```python
from build123d import *

# Parameters (mm, degrees)
RESSALTO_EXTRUS_O1_DEPTH = 12
RESSALTO_EXTRUS_O3_DEPTH = 6
ESBO_O4_W                = 3
ESBO_O4_H                = 26
RESSALTO_EXTRUS_O4_DEPTH = 22
ESBO_O6_W                = 2.5
ESBO_O6_H                = 9.5
RESSALTO_EXTRUS_O5_DEPTH = 2
ESBO_O7_R                = 1.1
CORTE_EXTRUS_O1_DEPTH    = 55.490824916
ESBO_O8_R                = 28.014084507
ESBO_O8_R_2              = 25.514084507
CORTE_EXTRUS_O2_DEPTH    = 3
FILETE1_R                = 1


with BuildPart() as part:
    # Esboço1 → Ressalto-extrusão1 (new body)
    with BuildSketch(Plane(origin=(0, 0, 0), x_dir=(1, 0, 0), z_dir=(0, 1, 0))):
        with BuildLine():
            Line((1.5, -16.431676725), (1.5, -13))
            Line((1.5, -13), (-0.5, -13))
            Line((-0.5, -13), (-0.5, 13))
            Line((-0.5, 13), (1.5, 13))
            Line((1.5, 13), (1.5, 16.431676725))
            ThreePointArc((1.5, 16.431676725), (6.342987532, 15.232088142), (10.60599556, 12.639733311))
            Line((10.60599556, 12.639733311), (13.819933608, 16.469955527))
            ThreePointArc((13.819933608, 16.469955527), (-21.5, 0), (13.819933608, -16.469955527))
            Line((13.819933608, -16.469955527), (10.60599556, -12.639733311))
            ThreePointArc((10.60599556, -12.639733311), (6.342987532, -15.232088142), (1.5, -16.431676725))
        make_face()
    extrude(amount=-RESSALTO_EXTRUS_O1_DEPTH)

    # Esboço3 → Ressalto-extrusão3 (add)
    with BuildSketch(Plane(origin=(0, 0, 0), x_dir=(1, 0, 0), z_dir=(0, 1, 0))):
        with BuildLine():
            Line((13.819933608, -16.469955527), (22.818960144, -27.194577731))
            ThreePointArc((22.818960144, -27.194577731), (-35.5, 0), (22.818960144, 27.194577731))
            Line((22.818960144, 27.194577731), (13.819933608, 16.469955527))
            ThreePointArc((13.819933608, 16.469955527), (-21.5, 0), (13.819933608, -16.469955527))
        make_face()
    extrude(amount=-RESSALTO_EXTRUS_O3_DEPTH)

    # Esboço4 → Ressalto-extrusão4 (add)
    with BuildSketch(Plane(origin=(0, 0, 0), x_dir=(1, 0, 0), z_dir=(0, 1, 0))):
        with Locations((-2, 0)):
            Rectangle(ESBO_O4_W, ESBO_O4_H)
    extrude(amount=RESSALTO_EXTRUS_O4_DEPTH)

    # Esboço6 → Ressalto-extrusão5 (add)
    with BuildSketch(Plane(origin=(-0.5, 0, 0), x_dir=(0, 0, -1), z_dir=(1, 0, 0))):
        with Locations((-11.75, -7.25)):
            Rectangle(ESBO_O6_W, ESBO_O6_H)
        with Locations((11.75, -7.25)):
            Rectangle(ESBO_O6_W, ESBO_O6_H)
    extrude(amount=RESSALTO_EXTRUS_O5_DEPTH)

    # Esboço7 → Corte-extrusão1 (cut, through all)
    with BuildSketch(Plane(origin=(-0.5, 0, 0), x_dir=(0, 0, -1), z_dir=(1, 0, 0))):
        with Locations((-10.4, 19.5)):
            Circle(ESBO_O7_R)
        with Locations((10.4, 19.5)):
            Circle(ESBO_O7_R)
        with Locations((10.4, 7)):
            Circle(ESBO_O7_R)
        with Locations((-10.4, 7)):
            Circle(ESBO_O7_R)
    extrude(amount=-CORTE_EXTRUS_O1_DEPTH, mode=Mode.SUBTRACT)

    # Esboço8 → Corte-extrusão2 (cut)
    with BuildSketch(Plane(origin=(0, 0, 0), x_dir=(1, 0, 0), z_dir=(0, 1, 0))):
        Circle(ESBO_O8_R)
        Circle(ESBO_O8_R_2, mode=Mode.SUBTRACT)
    extrude(amount=-CORTE_EXTRUS_O2_DEPTH, mode=Mode.SUBTRACT)

    # Filete1
    # the kernel refuses this fillet: 1 mm, written as the material it takes off along each edge
    with BuildSketch(Plane(origin=(-2.5, 21, 12), x_dir=(0, 0, 1), z_dir=(-1, 0, 0))) as filete1_piece_1_section:
        Polygon((0, 0), (FILETE1_R * 1.02, 0), (FILETE1_R * 1.02, FILETE1_R * 1.02), (0, FILETE1_R * 1.02), align=None)
    filete1_piece_1 = extrude(amount=FILETE1_R * 1.02, mode=Mode.PRIVATE)
    filete1_piece_1 = filete1_piece_1 - Plane(origin=(-2.5, 21, 12), x_dir=(0, -0.7071067811865475, -0.7071067811865475), z_dir=(-1, 0, 0)) * Sphere(FILETE1_R, mode=Mode.PRIVATE)
    add(filete1_piece_1, mode=Mode.SUBTRACT)
    with BuildSketch(Plane(origin=(-1.5, 21, 12), x_dir=(0, 0, 1), z_dir=(0, 1, 0))) as filete1_piece_2_section:
        Polygon((0, 0), (FILETE1_R * 1.02, 0), (FILETE1_R * 1.02, FILETE1_R * 1.02), (0, FILETE1_R * 1.02), align=None)
    filete1_piece_2 = extrude(amount=FILETE1_R * 1.02, mode=Mode.PRIVATE)
    filete1_piece_2 = filete1_piece_2 - Plane(origin=(-1.5, 21, 12), x_dir=(-0.7071067811865476, 0, -0.7071067811865475), z_dir=(0, 1, 0)) * Sphere(FILETE1_R, mode=Mode.PRIVATE)
    add(filete1_piece_2, mode=Mode.SUBTRACT)
    with BuildSketch(Plane(origin=(-1.5, 21, -12), x_dir=(1, 0, 0), z_dir=(0, 1, 0))) as filete1_piece_3_section:
        Polygon((0, 0), (FILETE1_R * 1.02, 0), (FILETE1_R * 1.02, FILETE1_R * 1.02), (0, FILETE1_R * 1.02), align=None)
    filete1_piece_3 = extrude(amount=FILETE1_R * 1.02, mode=Mode.PRIVATE)
    filete1_piece_3 = filete1_piece_3 - Plane(origin=(-1.5, 21, -12), x_dir=(-0.7071067811865475, 0, 0.7071067811865477), z_dir=(0, 1, 0)) * Sphere(FILETE1_R, mode=Mode.PRIVATE)
    add(filete1_piece_3, mode=Mode.SUBTRACT)
    with BuildSketch(Plane(origin=(-2.5, 21, -12), x_dir=(0, 1, 0), z_dir=(-1, 0, 0))) as filete1_piece_4_section:
        Polygon((0, 0), (FILETE1_R * 1.02, 0), (FILETE1_R * 1.02, FILETE1_R * 1.02), (0, FILETE1_R * 1.02), align=None)
    filete1_piece_4 = extrude(amount=FILETE1_R * 1.02, mode=Mode.PRIVATE)
    filete1_piece_4 = filete1_piece_4 - Plane(origin=(-2.5, 21, -12), x_dir=(0, -0.7071067811865475, 0.7071067811865475), z_dir=(-1, 0, 0)) * Sphere(FILETE1_R, mode=Mode.PRIVATE)
    add(filete1_piece_4, mode=Mode.SUBTRACT)
    with BuildSketch(Plane(origin=(1.5, 0, -10.5), x_dir=(-1, 0, 0), z_dir=(0, 0, -1))) as filete1_piece_5_section:
        with BuildLine():
            CenterArc((FILETE1_R, -FILETE1_R), FILETE1_R, 90, 90)
            Line((0, -FILETE1_R), (0, 0))
            Line((0, 0), (FILETE1_R, 0))
        make_face()
    filete1_piece_5 = extrude(amount=8.431676725, mode=Mode.PRIVATE)
    filete1_piece_5 = filete1_piece_5 & Plane(origin=(0, 0, 0), x_dir=(0.09090909090909027, 0, -0.9958591954639385), z_dir=(0, 1, 0)) * Cylinder(16.5, 21, mode=Mode.PRIVATE)
    add(filete1_piece_5, mode=Mode.SUBTRACT)
    with BuildSketch(Plane(origin=(0, 0, 0), x_dir=(0.7087130276081794, 0, -0.7054968777382703), z_dir=(0.7054968777382703, 0, 0.7087130276081794))) as filete1_piece_6:
        with BuildLine():
            CenterArc((28.014084507 + FILETE1_R, -FILETE1_R), FILETE1_R, 90, 90)
            Line((28.014084507, -FILETE1_R), (28.014084507, 0))
            Line((28.014084507, 0), (28.014084507 + FILETE1_R, 0))
        make_face()
    revolve(axis=Axis((0, 0, 0), (0, 1, 0)), revolution_arc=270.260599923, mode=Mode.SUBTRACT)
    with BuildSketch(Plane(origin=(1.5, 0, 18.931676725), x_dir=(-1, 0, 0), z_dir=(0, 0, -1))) as filete1_piece_7_section:
        with BuildLine():
            CenterArc((FILETE1_R, -FILETE1_R), FILETE1_R, 90, 90)
            Line((0, -FILETE1_R), (0, 0))
            Line((0, 0), (FILETE1_R, 0))
        make_face()
    filete1_piece_7 = extrude(amount=8.431676725, mode=Mode.PRIVATE)
    filete1_piece_7 = filete1_piece_7 & Plane(origin=(0, 0, 0), x_dir=(0.6427876096865377, 0, 0.7660444431189795), z_dir=(0, 1, 0)) * Cylinder(16.5, 21, mode=Mode.PRIVATE)
    add(filete1_piece_7, mode=Mode.SUBTRACT)
    with BuildSketch(Plane(origin=(0, 0, 0), x_dir=(0.7510532880617147, 0, 0.6602415910041466), z_dir=(0.6602415910041466, 0, -0.7510532880617147))) as filete1_piece_8_section:
        with BuildLine():
            CenterArc((16.5 + FILETE1_R, FILETE1_R), FILETE1_R, 180, 90)
            Line((16.5, FILETE1_R), (16.5, 0))
            Line((16.5, 0), (16.5 + FILETE1_R, 0))
        make_face()
    filete1_piece_8 = revolve(axis=Axis((0, 0, 0), (0, -1, 0)), revolution_arc=52.147490436, mode=Mode.PRIVATE)
    filete1_piece_8 = split(filete1_piece_8, bisect_by=Plane(origin=(1.5, 0, 0), z_dir=(1, 0, 0)), keep=Keep.TOP, mode=Mode.PRIVATE)
    add(filete1_piece_8, mode=Mode.SUBTRACT)
    with BuildSketch(Plane(origin=(0, 0, 0), x_dir=(0.6952666452885745, 0, 0.7187518987447418), z_dir=(0.7187518987447418, 0, -0.6952666452885745))) as filete1_piece_9:
        with BuildLine():
            CenterArc((35.5 - FILETE1_R, FILETE1_R), FILETE1_R, 270, 90)
            Line((35.5 - FILETE1_R, 0), (35.5, 0))
            Line((35.5, 0), (35.5, FILETE1_R))
        make_face()
    revolve(axis=Axis((0, 0, 0), (0, -1, 0)), revolution_arc=268.096938404, mode=Mode.SUBTRACT)
    with BuildSketch(Plane(origin=(-3.5, 0, 13), x_dir=(0, 0, -1), z_dir=(0, 1, 0)), Plane(origin=(-0.5, 0, 13), x_dir=(-1, 0, 0), z_dir=(0, 1, 0)), Plane(origin=(-3.5, 0, -13), x_dir=(1, 0, 0), z_dir=(0, 1, 0))) as filete1_piece_10:
        with BuildLine():
            CenterArc((FILETE1_R, -FILETE1_R), FILETE1_R, 90, 90)
            Line((0, -FILETE1_R), (0, 0))
            Line((0, 0), (FILETE1_R, 0))
        make_face()
    extrude(amount=21, mode=Mode.SUBTRACT)
    with BuildSketch(Plane(origin=(-0.5, 0, -13), x_dir=(-1, 0, 0), z_dir=(0, 1, 0))) as filete1_piece_11:
        with BuildLine():
            CenterArc((FILETE1_R, FILETE1_R), FILETE1_R, 180, 90)
            Line((0, FILETE1_R), (0, 0))
            Line((0, 0), (FILETE1_R, 0))
        make_face()
    extrude(amount=21, mode=Mode.SUBTRACT)
    with BuildSketch(Plane(origin=(-2.5, 22, 13), x_dir=(0, -1, 0), z_dir=(1, 0, 0)), Plane(origin=(-1.5, 22, -13), x_dir=(0, -1, 0), z_dir=(-1, 0, 0))) as filete1_piece_12:
        with BuildLine():
            CenterArc((FILETE1_R, FILETE1_R), FILETE1_R, 180, 90)
            Line((0, FILETE1_R), (0, 0))
            Line((0, 0), (FILETE1_R, 0))
        make_face()
    extrude(amount=1, mode=Mode.SUBTRACT)
    with BuildSketch(Plane(origin=(-0.5, 22, 12), x_dir=(0, -1, 0), z_dir=(0, 0, -1)), Plane(origin=(-3.5, 22, -12), x_dir=(0, -1, 0), z_dir=(0, 0, 1))) as filete1_piece_13:
        with BuildLine():
            CenterArc((FILETE1_R, FILETE1_R), FILETE1_R, 180, 90)
            Line((0, FILETE1_R), (0, 0))
            Line((0, 0), (FILETE1_R, 0))
        make_face()
    extrude(amount=24, mode=Mode.SUBTRACT)
    with BuildSketch(Plane(origin=(1.5, 0, 18.931676725), x_dir=(-1, 0, 0), z_dir=(0, 0, -1))) as filete1_piece_14a_section:
        with BuildLine():
            CenterArc((FILETE1_R, -FILETE1_R), FILETE1_R, 90, 90)
            Line((0, -FILETE1_R), (0, 0))
            Line((0, 0), (FILETE1_R, 0))
        make_face()
    filete1_piece_14a = extrude(amount=5.931676725, mode=Mode.PRIVATE)
    filete1_piece_14a = filete1_piece_14a - Plane(origin=(0, 0, 0), x_dir=(0.6427876096865377, 0, 0.7660444431189795), z_dir=(0, 1, 0)) * Cylinder(16.5, 16, mode=Mode.PRIVATE)
    with BuildSketch(Plane(origin=(0, 0, 0), x_dir=(0.6427876096865377, 0, 0.7660444431189793), z_dir=(0.7660444431189793, 0, -0.6427876096865377))) as filete1_piece_14b_section:
        with BuildLine():
            CenterArc((16.5 + FILETE1_R, FILETE1_R), FILETE1_R, 180, 90)
            Line((16.5, FILETE1_R), (16.5, 0))
            Line((16.5, 0), (16.5 + FILETE1_R, 0))
        make_face()
    filete1_piece_14b = revolve(axis=Axis((0, 0, 0), (0, -1, 0)), revolution_arc=43.465790933, mode=Mode.PRIVATE)
    filete1_piece_14b = split(filete1_piece_14b, bisect_by=Plane(origin=(1.5, 0, 0), z_dir=(-1, 0, 0)), keep=Keep.TOP, mode=Mode.PRIVATE)
    filete1_piece_14 = filete1_piece_14a & filete1_piece_14b
    add(filete1_piece_14, mode=Mode.SUBTRACT)


solid = part.part
```
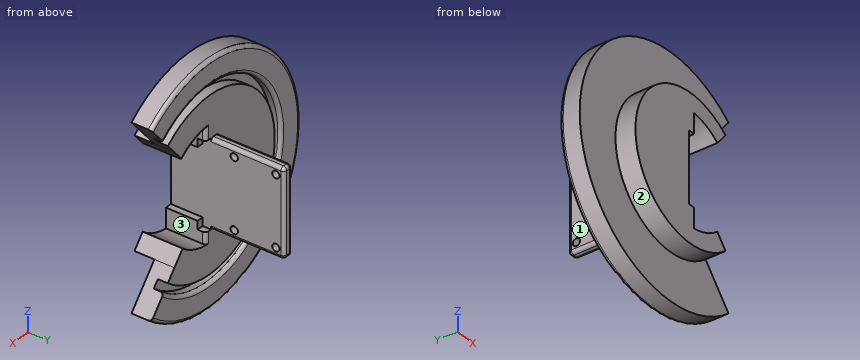
Verification items for the finished model (mm, model axes). Face numbers are marked on the shaded views. Round coordinates to 2 decimals unless told otherwise and drop trailing zeros. Order: outer loops, then holes, each group sorted by start corner. A loop starts at its lowest first (then second) coordinate and runs counter-clockwise, first axis right, second up. Notation, with made-up numbers: (73.25, -6) - (114.25, -6) arc R22 cw to (114.25, 24) - close; hole circle Ø3 at (-32.5, 37). An arc over 180 degrees is marked (long way). Use CSV: the item, a comma, the result in double quotes.
(1) Section check A-A on y = 19.5. Record the boundary of the cut face in (x, z).
Entries:
outline,"(-3.5, -12) arc R1 ccw to (-2.5, -13) - (-1.5, -13) arc R1 ccw to (-0.5, -12) - (-0.5, -11.5) - (-3.5, -11.5) - close; (-3.5, -9.3) - (-0.5, -9.3) - (-0.5, 9.3) - (-3.5, 9.3) - close; (-3.5, 11.5) - (-0.5, 11.5) - (-0.5, 12) arc R1 ccw to (-1.5, 13) - (-2.5, 13) arc R1 ccw to (-3.5, 12) - close"
(2) Section check C-C on y = 16. Record the boundary of the cut face in (x, z).
Entries:
outline,"(-3.5, -12) arc R1 ccw to (-2.5, -13) - (-1.5, -13) arc R1 ccw to (-0.5, -12) - (-0.5, 12) arc R1 ccw to (-1.5, 13) - (-2.5, 13) arc R1 ccw to (-3.5, 12) - close"
(3) Gauge pin test, flat ends, axial feed: pin 1 Ø2 at (x, z) = (0, -12) entering from +Y; pin 2 Ø0.6 at (x, z) = (0.5, 11.5) entering from +Y; pin 3 Ø1 at (x, y) = (0, -1) entering from +Z. Record the tip position at first contact, or that the pin passes through.
Entries:
pin 1,"y = 21.87"
pin 2,"y = -2.5"
pin 3,"z = 35.5"
(4) Mould release check, pull along Z, two halves, no side actions. Record for the marked faces 1, 2 and 3: released by +Z, released by -Z, zero draft, split by the parting line, or undercut.
Entries:
face 1,"zero draft"
face 2,"split by the parting line"
face 3,"undercut"
(5) Section check B-B on y = -7.5. Record the boundary of the cut face in (x, z).
Entries:
outline,"(-0.5, -10.5) - (-0.5, 10.5) - (1.5, 10.5) - (1.5, 16.43) arc R16.5 cw to (10.61, 12.64) - (13.82, 16.47) arc R21.5 ccw (long way) to (13.82, -16.47) - (10.61, -12.64) arc R16.5 cw to (1.5, -16.43) - (1.5, -10.5) - close"
(6) Thickness scan on probe 1 along Z at (x, y) = (0, -1.7); probe 2 along Y at (x, z) = (-2, 10.4); probe 3 along Y at (x, z) = (-2, -10). Record the ranges inside material, lowest first. Write a range as from..to.
Entries:
probe 1,"-35.5..-28.01, -25.51..-13, 13..25.51, 28.01..35.5"
probe 2,"-12..5.9, 8.1..18.4, 20.6..22"
probe 3,"-12..5.98, 8.02..18.48, 20.52..22"
